```python
from build123d import *

# Parameters (mm, degrees)
SKETCH1_R           = 37.5
SKETCH1_R_2         = 25
BOSS_EXTRUDE1_DEPTH = 100
BOSS_EXTRUDE2_START = 30
SKETCH2_R           = 37.5
BOSS_EXTRUDE2_DEPTH = 1000
FILLET1_R           = 10


with BuildPart() as part:
    # Sketch1 → Boss-Extrude1 (new body)
    with BuildSketch(Plane.XY):
        Circle(SKETCH1_R)
        Circle(SKETCH1_R_2, mode=Mode.SUBTRACT)
    extrude(amount=BOSS_EXTRUDE1_DEPTH)

    # Sketch2 → Boss-Extrude2 (add)
    with BuildSketch(Plane(origin=(0, 0, 0), x_dir=(1, 0, 0), z_dir=(0, 1, 0)).offset(BOSS_EXTRUDE2_START)):
        with Locations(Location((0, -50, 0), (0, 0, 53.130102354))):
            Circle(SKETCH2_R)
    extrude(amount=BOSS_EXTRUDE2_DEPTH)

    # Fillet1
    # the kernel refuses this fillet: 10 mm, written as the material it adds along each edge
    with BuildSketch(Plane(origin=(22.5, 30, 131.460549623), x_dir=(0.6295317231300945, -0.7769747805256321, 0), z_dir=(0, 0, -1))) as fillet1_piece_1_section:
        with BuildLine():
            CenterArc((20.728167196, -9.698102468), FILLET1_R, 104.114519992, 114.90106237)
            Line((12.958419391, -15.993419699), (0, 0))
            ThreePointArc((0, 0), (9.144779645, -1.132115744), (18.289559291, 0))
        make_face()
    fillet1_piece_1 = extrude(amount=162.921099245, mode=Mode.PRIVATE)
    fillet1_piece_1 = fillet1_piece_1 & Plane(origin=(0, 26.517376083, 50), x_dir=(0.6000000000021779, 0, -0.7999999999983666), z_dir=(0, -1, 0)) * Cylinder(37.5, 400, mode=Mode.PRIVATE)
    add(fillet1_piece_1)
    with BuildSketch(Plane(origin=(-22.5, 30, 131.460549623), x_dir=(-0.6295317231300945, -0.7769747805256321, 0), z_dir=(0, 0, -1))) as fillet1_piece_2_section:
        with BuildLine():
            CenterArc((20.728167196, 9.698102468), FILLET1_R, 140.984417638, 114.90106237)
            Line((12.958419391, 15.993419699), (0, 0))
            ThreePointArc((0, 0), (9.144779645, 1.132115744), (18.289559291, 0))
        make_face()
    fillet1_piece_2 = extrude(amount=162.921099245, mode=Mode.PRIVATE)
    fillet1_piece_2 = fillet1_piece_2 & Plane(origin=(0, 26.517339573, 50), x_dir=(0.6000000000021779, 0, -0.7999999999983666), z_dir=(0, -1, 0)) * Cylinder(37.5, 400, mode=Mode.PRIVATE)
    add(fillet1_piece_2)


solid = part.part
```
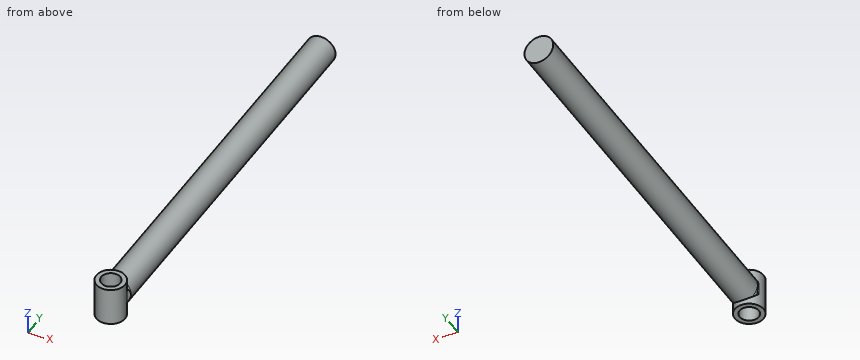
Model file for the job. Use its own axes, mm. Round coordinates to 2 decimals unless told otherwise and drop trailing zeros. Order: outer loops, then holes, each group sorted by start corner. A loop starts at its lowest first (then second) coordinate and runs counter-clockwise, first axis right, second up. Notation, with made-up numbers: M -29.5,-6 L -12.5,-6 A9 ccw -12.5,6 Z; hole C 36.25,68.5 d9. An arc over 180 degrees is marked long. Use CSV: the item, a comma, the result in double quotes.
Item 1: Saw through at D-D (y = 182). List the corners of the cut face in (x, z), plus the area to 3 significant figures.
Worked answers:
outline,"C 0,50 d75"
area,"4,420 mm²"
Item 2: Probe probe 1 along Y at (x, z) = (0, 67); probe 2 along Y at (x, z) = (14, 54); probe 3 along X at (y, z) = (862, 52). List the from-to ranges inside material, lowest first.
Worked answers:
probe 1,"-37.5 to -25, 25 to 1030"
probe 2,"-34.79 to -20.71, 20.71 to 1030"
probe 3,"-37.45 to 37.45"
Item 3: Saw through at C-C (z = 50). List the corners of the cut face in (x, y).
Worked answers:
outline,"M -37.5,28.3 A10 cw -34.01,15.79 A37.5 ccw long 34.01,15.79 A10 cw 37.5,28.3 L 37.5,1030 L -37.5,1030 Z; hole C 0,0 d50"
Item 4: Saw through at A-A (x = 0). List the corners of the cut face in (y, z), plus the area to 3 significant figures.
Worked answers:
outline,"M -37.5,0 L -25,0 L -25,100 L -37.5,100 Z; M 25,0 L 37.5,0 L 37.5,12.5 L 1030,12.5 L 1030,87.5 L 37.5,87.5 L 37.5,100 L 25,100 Z"
area,"76,900 mm²"
Item 5: Saw through at B-B (y = 0). List the corners of the cut face in (x, z).
Worked answers:
outline,"M -37.5,0 L -25,0 L -25,100 L -37.5,100 Z; M 25,0 L 37.5,0 L 37.5,100 L 25,100 Z"
Item 6: Pin check, flat tips, straight feed: pin 1 (4 mm diameter, centred on x = 26.5, y = 397, fed in from +Z); pin 2 (3 mm diameter, centred on x = 19.5, y = 709.5, fed in from +Z); pin 3 (4 mm diameter, centred on y = 257.5, z = 41, fed in from -X). Stop position of each tip, or through.
Worked answers:
pin 1,"z = 78.39"
pin 2,"z = 82.9"
pin 3,"x = -36.84"
